Build history of the part. All positions in model axes, mm. A direction names the side the tool comes from. Round coordinates to 2 decimals unless told otherwise and drop trailing zeros. Write each loop counter-clockwise with the first axis right and the second up, starting at its lowest first coordinate (ties: lowest second). Pieces come first, ordered by that corner, then holes.
Item 1: Wall check: probe 1 along Z at (x, y) = (-69.5, -38.1); probe 2 along Y at (x, z) = (-35.5, 25); probe 3 along Z at (x, y) = (-79.5, -51). Give the ranges that are in metal, low to high.
Item 2: Band-saw the part on C-C, the plane z = 45.5. Write the cut outline in (x, y), then the cut area to 3 significant figures.
Item 3: 3-axis set-ups, long thin cutter, end or side, ignore diameter. For faces 1 (the flat face through (-89, -6, 77.807)), 2 (the flat face through (-89, -38, 49.299)), 3 (the flat face through (-39.25, -32.1, 24.3)): which of +Z, -Z, +X, -X, +Y, -Y reach the whole face in a straight line?
Item 4: Band-saw the part on B-B, the plane x = -55. Write the cut outline in (y, z).
Item 5: Drop flat-ended pins along their axis: pin 1 Ø10 at (y, z) = (-48.5, 33.5) entering from +X; pin 2 Ø6 at (x, y) = (-108.5, -22) entering from +Z; pin 3 Ø12 at (y, z) = (-52.5, 27) entering from +X. Give the stop position or say it passes through.
Item 6: Band-saw the part on A-A, the plane y = -38.1. Write the cut outline in (x, z).
Item 7: Band-saw the part on D-D, the plane y = -23. Write the cut outline in (x, z), then the cut area to 3 significant figures.
```python
from build123d import *

# Parameters (mm, degrees)
F1_DEPTH = 12.7
F3_DEPTH = 50.8
F4_R     = 4.623587
F5_DEPTH = 120.853254


with BuildPart() as f1:
    # F0 (on Front) → F1 (new body)
    with BuildSketch(Plane.XZ):
        Polygon((-120.852254, 0), (0, 0), (-57.827156, 77.806771), (-120.852254, 77.806771), align=None)
    extrude(amount=F1_DEPTH)

    # F2 (on face) → F3 (join)
    with BuildSketch(Plane.XZ.offset(12.7)):
        Polygon((-57.827156, 49.29851), (-120.852254, 49.29851), (-120.852254, 0), (-21.187766, 0), align=None)
    extrude(amount=F3_DEPTH)

    # F4 (on face) → F5 (cut, through all)
    with BuildSketch(Plane(origin=(-120.852254, 0, 0), x_dir=(0, -1, 0), z_dir=(-1, 0, 0))):
        with Locations((38.1, 24.649255)):
            Circle(F4_R)
    extrude(amount=-F5_DEPTH, mode=Mode.SUBTRACT)


solid = f1.part
```
Results:
1. probe 1: z = 0 to 20.03, 29.27 to 49.3
1. probe 2: y = -12.7 to 0
1. probe 3: z = 0 to 49.3
2. outline: (-120.85, -63.5) - (-55, -63.5) - (-55, -12.7) - (-33.82, -12.7) - (-33.82, 0) - (-120.85, 0) - close
2. area: 4,450 mm2
3. face 1: +Z, +X, -X, +Y, -Y
3. face 2: +Z, +X, -X, -Y
3. face 3: +Z, +X, -Y
4. outline: (-63.5, 0) - (0, 0) - (0, 74) - (-12.7, 74) - (-12.7, 45.49) - (-63.5, 45.49) - close; hole circle Ø9.25 at (-38.1, 24.65)
5. pin 1: stops at x = -42.37
5. pin 2: stops at z = 49.3
5. pin 3: stops at x = -36.8
6. outline: (-120.85, 0) - (-21.19, 0) - (-36.07, 20.03) - (-120.85, 20.03) - close; (-120.85, 29.27) - (-42.94, 29.27) - (-57.83, 49.3) - (-120.85, 49.3) - close
7. outline: (-120.85, 0) - (-21.19, 0) - (-57.83, 49.3) - (-120.85, 49.3) - close
7. area: 4,010 mm2
